```python
from build123d import *

# Parameters (mm, degrees)
F0_W     = 40
F0_H     = 40
F1_DEPTH = 265
F2_W     = 20
F2_H     = 40
F3_DEPTH = 40
F5_DEPTH = 20


with BuildPart() as f1:
    # F0 (on Right) → F1 (new body)
    with BuildSketch(Plane.YZ):
        with Locations((-3.228404, 8.187629)):
            Rectangle(F0_W, F0_H)
    extrude(amount=F1_DEPTH)

    # F2 (on face) → F3 (join)
    with BuildSketch(Plane.YZ.offset(265)):
        with Locations((-3.228404, 8.187629)):
            Rectangle(F2_W, F2_H)
    extrude(amount=F3_DEPTH)

    # F4 (on face) → F5 (cut)
    with BuildSketch(Plane.YZ.offset(305)):
        Polygon((6.771596, -1.812371), (-13.228404, 3.187629), (-13.228404, -11.812371), (6.771596, -11.812371), align=None)
        Polygon((-13.228404, 28.187629), (-13.228404, 13.187629), (6.771596, 18.187629), (6.771596, 28.187629), align=None)
    extrude(amount=-F5_DEPTH, mode=Mode.SUBTRACT)

    # F6: F1 across face


with BuildPart() as f1_1:
    add(f1.part)
    add(f1.part.mirror(Plane(origin=(0, -3.228404, 8.187629), x_dir=(0, 1, 0), z_dir=(-1, 0, 0))))


solid = f1_1.part
```
Work out the finished part from the listing and answer in its coordinate system (mm). A direction names the side the tool comes from. Round coordinates to 2 decimals unless told otherwise and drop trailing zeros. Loops run counter-clockwise (first coordinate to the right, second up) from the corner with the lowest first, then second, coordinate; pieces in that order, holes last.
(1) Find the intervals of material crossed by L1, parallel to X at y = 10, z = -8; L2, parallel to X at y = 0, z = 24.5; L3, parallel to Y at x = 276.5, z = 19.5, in increasing order.
Computed values:
L1: x = -265 to 265
L2: x = -285 to 285
L3: y = -13.23 to 6.77
(2) The part is cut by section A-A, the plane y = -1.5. Give the vertices of the cut face in (x, z).
Computed values:
outline: (-305, 0.26) - (-285, 0.26) - (-285, -11.81) - (285, -11.81) - (285, 0.26) - (305, 0.26) - (305, 16.12) - (285, 16.12) - (285, 28.19) - (-285, 28.19) - (-285, 16.12) - (-305, 16.12) - close
(3) Each of these flat-tipped pins is pushed along its axis until it touches: P1, Ø4.5, axis at y = -4.5, z = 21.5, coming from the -X side; P2, Ø11, axis at y = 13, z = 8.5, coming from the +X side; P3, Ø5, axis at y = -18, z = 13, coming from the -X side. Where does it stop, or does it pass through?
Computed values:
P1: stops at x = -285
P2: stops at x = 265
P3: stops at x = -265
(4) For faces 1 (the flat face through (285, -3, -6)), 2 (the flat face through (-295.14, -3.368, 15.653)), 3 (the flat face through (280, -13.228, 8)), determine the directions among +Z, -Z, +X, -X, +Y, -Y from which every point of the face is accessible in a straight line to the end or side of a thin tool.
Computed values:
face 1: -Z, +X, -Y
face 2: +Z, -X, -Y
face 3: +Z, -Z, +X, -Y
